Can you work these out from the model? Positions are in its coordinate system, mm. Face numbers are marked on the shaded views. A direction names the side the tool comes from. Give positions to 0.01 mm unless a question says otherwise; leave off trailing zeros. Order: outer loops, then holes, each group sorted by start corner. A loop starts at its lowest first (then second) coordinate and runs counter-clockwise, first axis right, second up. Notation, with made-up numbers: (16, 23) -> (50, 23) arc R30 cw to (50, 50) -> close; hole circle Ø9 at (40, 44.25). An arc over 180 degrees is marked (long way). Answer as CSV lines item,"result".
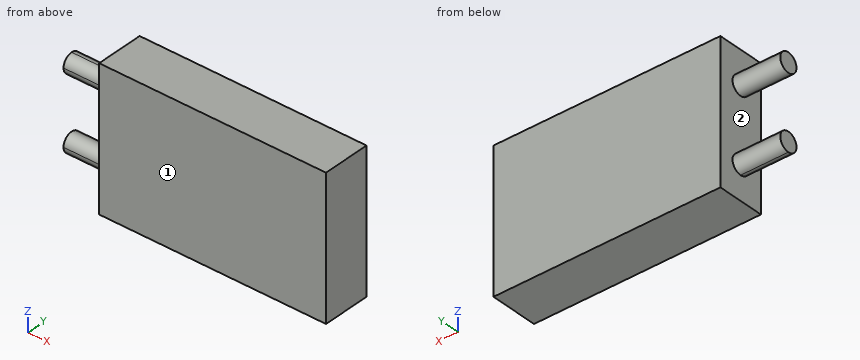
```python
from build123d import *

# Parameters (mm, degrees)
F0_W      = 60.33
F0_H      = 38.1
F1_DEPTH  = 12.7
F3_DEPTH  = 38.1
F4_W      = 11.2605243921
F4_H      = 14.8357795551
F5_DEPTH  = 3.175
F6_W      = 12.7
F6_H      = 0.254
F7_DEPTH  = 101.6
F8_W      = 7.62
F8_H      = 0.6586039143
F11_W     = 5.8358858012
F11_H     = 2.5163960857
F12_DEPTH = 7.62
F13_W     = 12.7
F13_H     = 0.508
F14_DEPTH = 101.6
F16_DEPTH = 17.78
F18_DEPTH = 25.4
F20_DEPTH = 12.7


with BuildPart() as f1:
    # F0 (on Front) → F1 (new body)
    with BuildSketch(Plane.XZ):
        with Locations((30.165, 19.05)):
            Rectangle(F0_W, F0_H)
    extrude(amount=F1_DEPTH)

    # F2 (on face) → F3 (join)
    with BuildSketch(Plane.XY.offset(38.1)):
        Polygon((0, -2.7734531851), (-7.62, 0), (-7.62, -12.7), (0, -9.9265468149), align=None)
    extrude(amount=-F3_DEPTH)

    # F4 (on face) → F5 (cut)
    with BuildSketch(Plane(origin=(0, 0, 0), x_dir=(1, 0, 0), z_dir=(0, 0, -1))):
        with Locations((-5.6302621961, 7.4178897776)):
            Rectangle(F4_W, F4_H)
    extrude(amount=-F5_DEPTH, mode=Mode.SUBTRACT)

    # F6 (on face) → F7 (cut)
    with BuildSketch(Plane.YZ.offset(60.33)):
        with Locations((-6.35, 37.973)):
            Rectangle(F6_W, F6_H)
    extrude(amount=-F7_DEPTH, mode=Mode.SUBTRACT)

    # F10: sweep along a path in F9
    with BuildLine(Plane(origin=(0, 0, 0), x_dir=(0, -1, 0), z_dir=(-1, 0, 0))) as f10_path:
        Line((2.7734531851, 3.175), (2.7734531851, 0))
        Line((2.7734531851, 0), (9.9265468149, 0))
        Line((9.9265468149, 0), (9.9265468149, 3.175))
    # F8 (on face) → F10 (sweep)
    with BuildSketch(Plane(origin=(0, 0, 3.175), x_dir=(1, 0, 0), z_dir=(0, 0, -1))):
        with Locations((-3.81, 3.1027551423)):
            Rectangle(F8_W, F8_H)
        Polygon((-7.62, 0), (0, 2.7734531851), (-7.62, 2.7734531851), align=None)
    sweep(path=f10_path.line, transition=Transition.RIGHT)

    # F11 (on face) → F12 (join)
    with BuildSketch(Plane(origin=(-7.62, 0, 0), x_dir=(0, -1, 0), z_dir=(-1, 0, 0))):
        with Locations((6.35, 1.9168019572)):
            Rectangle(F11_W, F11_H)
    extrude(amount=-F12_DEPTH)

    # F13 (on face) → F14 (cut)
    with BuildSketch(Plane.YZ.offset(60.33)):
        with Locations((-6.35, 37.592)):
            Rectangle(F13_W, F13_H)
    extrude(amount=-F14_DEPTH, mode=Mode.SUBTRACT)

    # F15 (on face) → F16 (cut)
    with BuildSketch(Plane.XY.offset(37.338)):
        Polygon((0, -2.7734531851), (-7.62, 0), (-7.62, -12.7), (0, -9.9265468149), align=None)
    extrude(amount=-F16_DEPTH, mode=Mode.SUBTRACT)

    # F17 (on face) → F18 (cut)
    with BuildSketch(Plane.XY.offset(19.558)):
        Polygon((-7.62, 0), (-7.62, -12.7), (0, -9.9265468149), (0, -2.7734531851), align=None)
    extrude(amount=-F18_DEPTH, mode=Mode.SUBTRACT)

    # F19 (on face) → F20 (join)
    with BuildSketch(Plane(origin=(0, 0, 0), x_dir=(0, -1, 0), z_dir=(-1, 0, 0))):
        with BuildLine():
            ThreePointArc((8.89, 8.89), (4.5539487758, 10.6860512242), (6.35, 6.35))
            ThreePointArc((6.35, 6.35), (8.1460512242, 7.0939487758), (8.89, 8.89))
        make_face()
        with BuildLine():
            ThreePointArc((8.89, 28.448), (8.1460512242, 30.2440512242), (6.35, 30.988))
            ThreePointArc((6.35, 30.988), (4.5539487758, 26.6519487758), (8.89, 28.448))
        make_face()
    extrude(amount=F20_DEPTH)


solid = f1.part
```
Item 1: Imagine slicing it at A-A, the plane y = -8. Please give me the cut outline in (x, z).
Numbers:
outline,"(-12.7, 6.96) -> (0, 6.96) -> (0, 0) -> (60.33, 0) -> (60.33, 37.34) -> (0, 37.34) -> (0, 30.38) -> (-12.7, 30.38) -> (-12.7, 26.52) -> (0, 26.52) -> (0, 10.82) -> (-12.7, 10.82) -> close"
Item 2: Imagine slicing it at C-C, the plane y = -1.75. Please give me the cut outline in (x, z), then the cut area to 3 significant figures.
Numbers:
outline,"(0, 0) -> (60.33, 0) -> (60.33, 37.34) -> (0, 37.34) -> close"
area,"2,250 mm²"
Item 3: For the marked faces 1 and 2, which set-ups out of +Z, -Z, +X, -X, +Y, -Y let a thin tool reach every point of the face, with its end or its side?
Numbers:
face 1,"+Z, -Z, +X, -X, -Y"
face 2,"-X"
Item 4: Please list where these lines run through material, in increasing order: line 1 along X through (y, z) = (-10, 24); line 2 along Z through (x, y) = (-6, -6); line 3 along Z through (x, y) = (-7.5, -7.75).
Numbers:
line 1,"x = 0 to 60.33"
line 2,"z = 6.37 to 11.41, 25.93 to 30.96"
line 3,"z = 6.77 to 11.01, 26.33 to 30.57"
Item 5: Imagine slicing it at B-B, the plane z = 20.5. Please give me the cut outline in (x, y), then the cut area to 3 significant figures.
Numbers:
outline,"(0, -12.7) -> (60.33, -12.7) -> (60.33, 0) -> (0, 0) -> close"
area,"766 mm²"
